Print and shaded views of the part. All mm, measured from the part's lowest x, y and z. A direction names the side the tool comes from. Round coordinates to 2 decimals unless told otherwise and drop trailing zeros. Loops run counter-clockwise (first coordinate to the right, second up) from the corner with the lowest first, then second, coordinate; pieces in that order, holes last. Notation, with made-up numbers: (57.25, 7) -> (110.25, 7) arc R27 cw to (110.25, 44) -> close; hole circle Ø11 at (-22, 84). An arc over 180 degrees is marked (long way). Use a Markdown table: item, result.
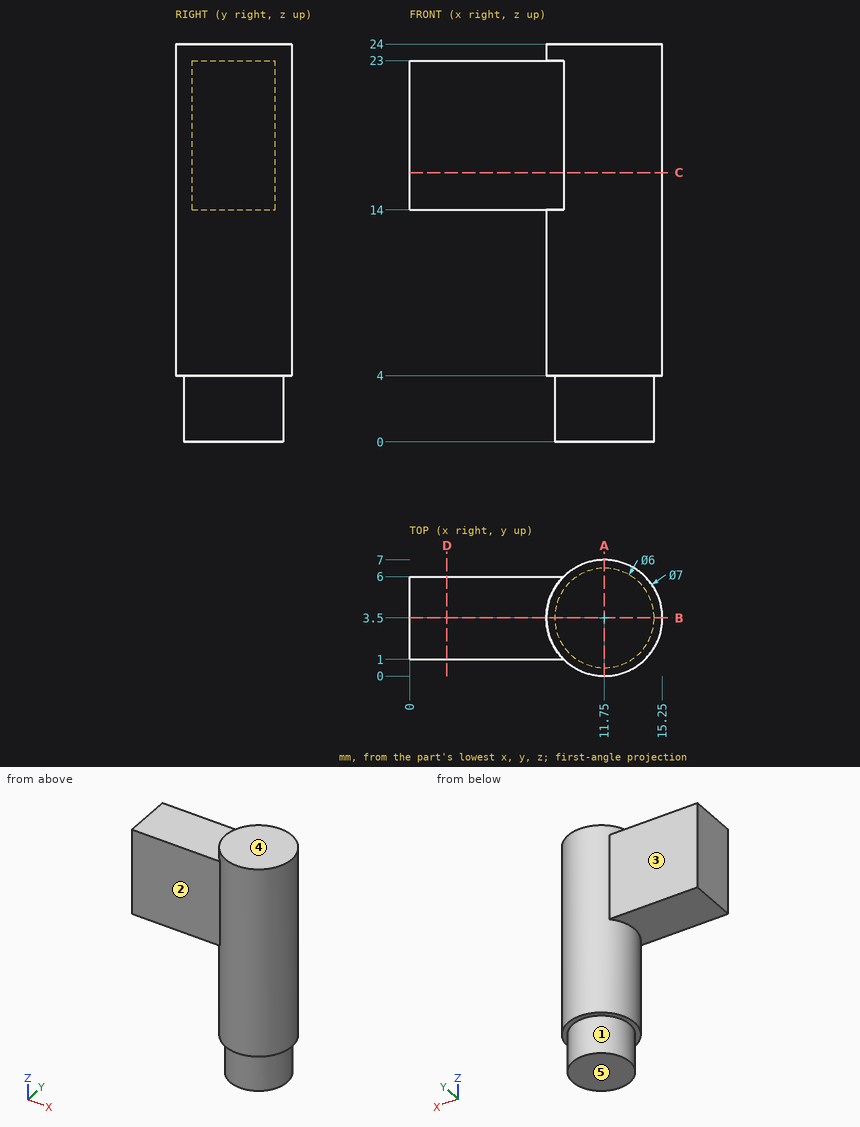
Q1. Flat gauge pins, fed straight in: pin 1 (2.5 mm diameter, centred on x = 3.5, y = 3, fed in from +Z); pin 2 (2 mm diameter, centred on y = 6, z = 18.5, fed in from -X); pin 3 (2.5 mm diameter, centred on x = 6.5, z = 20.5, fed in from +Y); pin 4 (2 mm diameter, centred on x = 4.5, y = 5.5, fed in from -Z). Where does each tip first touch, or does it go through?
Results list:
| item | result |
|---|---|
| pin 1 | stops at z = 23 |
| pin 2 | stops at x = 0 |
| pin 3 | stops at y = 6 |
| pin 4 | stops at z = 14 |
Q2. Band-saw the part on D-D, the plane x = 2.25. Give the cut face in (y, z), plus the area to 3 significant figures.
Results list:
| item | result |
|---|---|
| outline | (1, 14) -> (6, 14) -> (6, 23) -> (1, 23) -> close |
| area | 45.0 mm² |
Q3. Band-saw the part on C-C, the plane z = 16.25. Give the cut face in (x, y), plus the area to 3 significant figures.
Results list:
| item | result |
|---|---|
| outline | (0, 1) -> (9.3, 1) arc R3.5 ccw (long way) to (9.3, 6) -> (0, 6) -> close |
| area | 81.4 mm² |
Q4. Band-saw the part on B-B, the plane y = 3.5. Give the cut face in (x, z), plus the area to 3 significant figures.
Results list:
| item | result |
|---|---|
| outline | (0, 14) -> (8.25, 14) -> (8.25, 4) -> (8.75, 4) -> (8.75, 0) -> (14.75, 0) -> (14.75, 4) -> (15.25, 4) -> (15.25, 24) -> (8.25, 24) -> (8.25, 23) -> (0, 23) -> close |
| area | 238 mm² |
Q5. Drill centre lines: L1, parallel to X at y = 3.5, z = 12.75; L2, parallel to Z at x = 4.5, y = 2; L3, parallel to Y at x = 4.75, z = 20. Where is each one in solid material? Low to high. Write a range as from..to.
Results list:
| item | result |
|---|---|
| L1 | x = 8.25..15.25 |
| L2 | z = 14..23 |
| L3 | y = 1..6 |
Q6. Band-saw the part on A-A, the plane x = 11.75. Give the cut face in (y, z).
Results list:
| item | result |
|---|---|
| outline | (0, 4) -> (0.5, 4) -> (0.5, 0) -> (6.5, 0) -> (6.5, 4) -> (7, 4) -> (7, 24) -> (0, 24) -> close |
Q7. Tool access for the marked faces 1, 2, 3, 4 and 5: list every direction of +Z, -Z, +X, -X, +Y, -Y with a clear straight run to the whole face (end or side of a thin tool).
Results list:
| item | result |
|---|---|
| face 1 | -Z |
| face 2 | +Z, -Z, -X, -Y |
| face 3 | +Z, -Z, -X, +Y |
| face 4 | +Z, +X, -X, +Y, -Y |
| face 5 | -Z, +X, -X, +Y, -Y |
